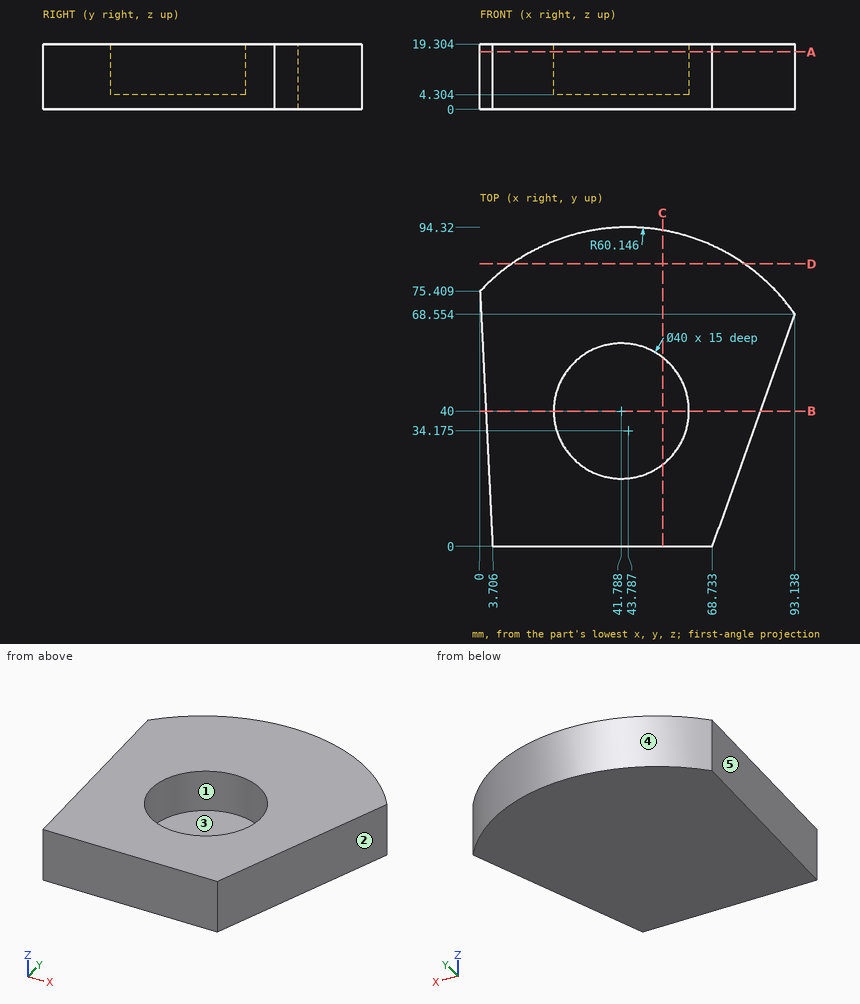
Job drawing, mm, ordinate dimensions from the low corner. One solid piece. A direction names the side the tool comes from. Coordinates: 2 decimals unless noted, no trailing zeros. Order: outer loops, then holes, each group sorted by start corner. A loop starts at its lowest first (then second) coordinate and runs counter-clockwise, first axis right, second up. Notation, with made-up numbers: (34.5, 58.5) -> (45.5, 58.5) arc R19 ccw to (45.5, 91.5) -> close; hole circle Ø6 at (-2.75, 14.5). An arc over 180 degrees is marked (long way). Return JSON: item names as keys, results as strings. Group by question number.
Item 1: Saw through at D-D on y = 83.5. Write the cut outline in (x, z).
Item 2: Tool access for the marked faces 1 and 2: list every direction of +Z, -Z, +X, -X, +Y, -Y with a clear straight run to the whole face (end or side of a thin tool).
Item 3: Flat gauge pins, fed straight in: P1, Ø1.5, axis at y = 58, z = 7.5, coming from the -X side; P2, Ø5, axis at y = 59.5, z = 9.5, coming from the -X side; P3, Ø6, axis at y = 65.5, z = 4.5, coming from the +X side. Where does each tip first touch, or does it go through?
Item 4: Wall check: line 1 along Y through (x, z) = (36, 15) (1 decimal); line 2 along X through (y, z) = (51, 7) (1 decimal); line 3 along Y through (x, z) = (44, 11.25). Give the ranges that are in metal, low to high. Write a range as [from, to].
Item 5: Saw through at A-A on z = 17. Write the cut outline in (x, y) (1 decimal), then the cut area to 3 significant figures.
Item 6: Saw through at C-C on x = 54. Write the cut outline in (y, z).
Item 7: Pull direction X, two halves, no side cores. Call the marked faces 3, 4 and 5: pulls with the +X half, pulls with the -X half, needs draft (parallel to the pull), parting line crosses it, or undercut.
Item 8: Saw through at B-B on y = 40. Write the cut outline in (x, z).
Values found:
{
 "1": {"outline": "(9.37, 0) -> (78.2, 0) -> (78.2, 19.3) -> (9.37, 19.3) -> close"},
 "2": {"face 1": "+Z", "face 2": "+Z, -Z, +X, -Y"},
 "3": {"P1": "stops at x = 0.82", "P2": "stops at x = 0.66", "P3": "stops at x = 93.12"},
 "4": {"line 1": "y = [0, 20.9], [59.1, 93.8]", "line 2": "x = [1.2, 25.1], [58.5, 86.9]", "line 3": "y = [0, 20.12], [59.88, 94.32]"},
 "5": {"outline": "(0, 75.4) -> (3.7, 0) -> (68.7, 0) -> (93.1, 68.6) arc R60.1 ccw to start; hole circle Ø40 at (41.8, 40)", "area": "5,920 mm2"},
 "6": {"outline": "(0, 0) -> (93.45, 0) -> (93.45, 19.3) -> (55.84, 19.3) -> (55.84, 4.3) -> (24.16, 4.3) -> (24.16, 19.3) -> (0, 19.3) -> close"},
 "7": {"face 3": "undercut", "face 4": "parting line crosses it", "face 5": "pulls with the -X half"},
 "8": {"outline": "(1.74, 0) -> (82.97, 0) -> (82.97, 19.3) -> (61.79, 19.3) -> (61.79, 4.3) -> (21.79, 4.3) -> (21.79, 19.3) -> (1.74, 19.3) -> close"}
}
